Autodesk Fusion 360 part; units mm, degrees
sketch "Sketch1" plane through (0, 0, 0) normal (0, 0, 1) x (1, 0, 0)
  line L0 (0, 0) -> (160, 0)
  line L1 (160, 0) -> (160, 160)
  line L2 (160, 160) -> (0, 160)
  line L3 (0, 160) -> (0, 0)
  dimension "d1" = 160
  dimension "d3" = 160
extrude "Extrude1" add sketch "Sketch1" along normal blind 30
fillet "Fillet1" radius 5 4 edges at (0, 160, 15) (0, 0, 15) (160, 0, 15) (160, 160, 15)
fillet "Fillet1" radius 3 4 edges at (160, 80, 30) (80, 160, 30) (80, 0, 30) (0, 80, 30)
shell "Shell1" thickness 2.7 removed faces 1 at (53.3333, 51.6667, 0)
sketch "Sketch3" plane through (0, 0, 30) normal (0, 0, 1) x (-1, 0, 0)
  arc A0 (-5, -157) -> (-3, -155) centre (-5, -155) ccw
  line L0 (-3, -155) -> (-3, -5)
  arc A1 (-3, -5) -> (-5, -3) centre (-5, -5) ccw
  line L1 (-5, -3) -> (-155, -3)
  arc A2 (-155, -3) -> (-157, -5) centre (-155, -5) ccw
  line L2 (-157, -5) -> (-157, -155)
  arc A3 (-157, -155) -> (-155, -157) centre (-155, -155) ccw
  line L3 (-155, -157) -> (-5, -157)
  line L4 (-44.5, -145) -> (-115.5, -145)
  line L5 (-115.5, -145) -> (-115.5, -118)
  line L6 (-115.5, -118) -> (-44.5, -118)
  line L7 (-44.5, -118) -> (-44.5, -145)
  arc A4 (-155, 0) -> (-160, -5) centre (-155, -5) ccw
  line L8 (-160, -5) -> (-160, -155)
  arc A5 (-160, -155) -> (-155, -160) centre (-155, -155) ccw
  line L9 (-155, -160) -> (-5, -160)
  arc A6 (-5, -160) -> (0, -155) centre (-5, -155) ccw
  line L10 (0, -155) -> (0, -5)
  arc A7 (0, -5) -> (-5, 0) centre (-5, -5) ccw
  line L11 (-5, 0) -> (-155, 0)
  line L12 (-80, -145) -> (-80, -160) construction
  dimension "d11" = 71
  dimension "d12" = 27
  dimension "d13" = 15
extrude "Extrude2" cut sketch "Sketch3" along normal through all and the other way through all contours L4 L5 L6 L7
sketch "Sketch4" plane through (0, 0, 30) normal (0, 0, 1) x (-1, 0, 0)
  line L0 (-44.5, -145) -> (-44.5, -118)
  line L1 (-44.5, -118) -> (-115.5, -118)
  line L2 (-115.5, -118) -> (-115.5, -145)
  line L3 (-115.5, -145) -> (-44.5, -145)
  arc A0 (-155, 0) -> (-160, -5) centre (-155, -5) ccw
  line L4 (-160, -5) -> (-160, -155)
  arc A1 (-160, -155) -> (-155, -160) centre (-155, -155) ccw
  line L5 (-155, -160) -> (-5, -160)
  arc A2 (-5, -160) -> (0, -155) centre (-5, -155) ccw
  line L6 (0, -155) -> (0, -5)
  arc A3 (0, -5) -> (-5, 0) centre (-5, -5) ccw
  line L7 (-5, 0) -> (-155, 0)
  line L8 (-37.5, -144) -> (-122.5, -144)
  line L9 (-122.5, -144) -> (-122.5, -119)
  line L10 (-122.5, -119) -> (-37.5, -119)
  line L11 (-37.5, -119) -> (-37.5, -144)
  line L12 (-44.5, -131.5) -> (-37.5, -131.5)
  line L13 (-80, -144) -> (-80, -145)
  line L14 (-80, -118) -> (-80, -119)
  line L15 (-115.5, -131.5) -> (-122.5, -131.5)
  dimension "d31" = 85
  dimension "d32" = 25
sketch "Sketch5" plane through (0, 0, 30) normal (0, 0, 1) x (-1, 0, 0)
  line L0 (-44.5, -118) -> (-44.5, -145)
  line L1 (-44.5, -145) -> (-115.5, -145)
  line L2 (-115.5, -145) -> (-115.5, -118)
  line L3 (-115.5, -118) -> (-44.5, -118)
  arc A0 (-5, -157) -> (-3, -155) centre (-5, -155) ccw
  line L4 (-3, -155) -> (-3, -5)
  arc A1 (-3, -5) -> (-5, -3) centre (-5, -5) ccw
  line L5 (-5, -3) -> (-155, -3)
  arc A2 (-155, -3) -> (-157, -5) centre (-155, -5) ccw
  line L6 (-157, -5) -> (-157, -155)
  arc A3 (-157, -155) -> (-155, -157) centre (-155, -155) ccw
  line L7 (-155, -157) -> (-5, -157)
  circle A4 centre (-45.0613, -144.4387) radius 0.7937
  line L8 (-44.5, -145) -> (-45.0613, -144.4387)
  circle A5 centre (-114.9387, -144.4387) radius 0.7937
  line L9 (-115.5, -145) -> (-114.9387, -144.4387) construction
  dimension "d23" = 1.5875
  dimension "d24" = 45
  dimension "d25" = 1.5875
extrude "Extrude3" [suppressed]
ref_plane "WorkPlane1" through (80, 131.5, 28.65) normal (0, -1, 0) x (-1, 0, 0)
mirror "Mirror1" [suppressed]
fillet "Fillet2" radius 0.793 4 edges at (44.5, 145, 28.65) (115.5, 145, 28.65) (115.5, 118, 28.65) (44.5, 118, 28.65)
hole "Hole1" at (122.5, 144, 30) at (122.5, 119, 30) at (37.5, 119, 30) at (37.5, 144, 30) direction (0, 0, -1) diameter 3.4 depth 15 tip angle 118 countersink diameter 7.5 countersink angle 90
equation "d1 = Lid_X"
equation "d3 = Lid_Y"
equation "d4 = Lid_Z"
equation "d8 = Lid_Thikness"
equation "d11 = Opening_X"
equation "d12 = Opening_Y"
equation "d23 = ( 1 / 16 ) * 1 in"
equation "d25 = 1 / 16 * 1 in"
equation "d30 = Corner_rad"
equation "d31 = Holes_X"
equation "d32 = Holes_Y"
equation "Lid_X = 160 mm"
equation "Lid_Y = 160 mm"
equation "Lid_Z = 30 mm"
equation "Opening_X = 71 mm"
equation "Opening_Y = 27 mm"
equation "Lid_Thikness = 2.7 mm"
equation "Corner_rad = 0.793 mm"
equation "Holes_X = 85 mm"
equation "Holes_Y = 25 mm"
Build history of the part. All positions in model axes, mm. A direction names the side the tool comes from. Give positions to 0.01 mm unless a question says otherwise; leave off trailing zeros. Order: outer loops, then holes, each group sorted by start corner. A loop starts at its lowest first (then second) coordinate and runs counter-clockwise, first axis right, second up. Notation, with made-up numbers: M 87.5,22 L 100.5,22 A33 cw 100.5,54 Z; hole C 6.5,1.5 d4. An arc over 180 degrees is marked long. Use one line per item in the form item = value.
1) Probe probe 1 along X at (y, z) = (119, 27.5); probe 2 along X at (y, z) = (20.5, 10.5). List the from-to ranges inside material, lowest first.
Calculated:
probe_1 = 0.04 to 35.8, 39.2 to 44.5, 115.5 to 120.8, 124.2 to 159.96
probe_2 = 0 to 2.7, 157.3 to 160
2) Saw through at B-B (z = 8). Give the cut face in (x, y), plus the area to 3 significant figures.
Calculated:
outline = M 0,5 A5 ccw 5,0 L 155,0 A5 ccw 160,5 L 160,155 A5 ccw 155,160 L 5,160 A5 ccw 0,155 Z; hole M 2.7,5 A2.3 ccw 5,2.7 L 155,2.7 A2.3 ccw 157.3,5 L 157.3,155 A2.3 ccw 155,157.3 L 5,157.3 A2.3 ccw 2.7,155 Z
area = 1,680 mm2
3) Drop flat-ended pins along their axis: pin 1 (4 mm diameter, centred on y = 99.5, z = 18.5, fed in from -X); pin 2 (3 mm diameter, centred on x = 37.5, y = 119, fed in from +Z); pin 3 (4 mm diameter, centred on x = 81, y = 47.5, fed in from -Z); pin 4 (1.3 mm diameter, centred on x = 95, z = 28, fed in from +Y). Give the stop position or say it passes through.
Calculated:
pin_1 = 0
pin_2 = through
pin_3 = 27.3
pin_4 = 159.98
4) Tool access for faces 4 (the face through (35.715, 119.396, 28.078)), 5 (the face through (81, 157.3, 13)): list every direction of +Z, -Z, +X, -X, +Y, -Y with a clear straight run to the whole face (end or side of a thin tool).
Calculated:
face_4 = +Z
face_5 = -Z
5) Saw through at C-C (x = 110.5). Give the cut face in (y, z), plus the area to 3 significant figures.
Calculated:
outline = M 0,0 L 2.7,0 L 2.7,27 A0.3 cw 3,27.3 L 118,27.3 L 118,30 L 3,30 A3 ccw 0,27 Z; M 145,27.3 L 157,27.3 A0.3 cw 157.3,27 L 157.3,0 L 160,0 L 160,27 A3 ccw 157,30 L 145,30 Z
area = 503 mm2
6) Two-plate mould, pull along Y, no slides. Class faces 1 (the face through (160, 79, 13)), 2 (the face through (81, 160, 13)), 3 (the face through (79, 2.7, 13)): released by +Y, released by -Y, zero draft, split by the parting line, or undercut.
Calculated:
face_1 = zero draft
face_2 = released by +Y
face_3 = undercut
7) Saw through at A-A (y = 61.5). Give the cut face in (x, z).
Calculated:
outline = M 0,0 L 2.7,0 L 2.7,27 A0.3 cw 3,27.3 L 157,27.3 A0.3 cw 157.3,27 L 157.3,0 L 160,0 L 160,27 A3 ccw 157,30 L 3,30 A3 ccw 0,27 Z
